Geometry: see drawing. Coordinates: mm, zero at the bounding-box minimum. A direction names the side the tool comes from. Give positions to 0.01 mm unless a question says otherwise; leave off trailing zeros. Order: outer loops, then holes, each group sorted by start corner. A loop starts at its lowest first (then second) coordinate and runs counter-clockwise, first axis right, second up. Notation, with made-up numbers: M 65,17.25 L 121,17.25 A22 cw 121,46.25 Z; hole C 29,-37.75 d11. An arc over 180 degrees is marked long. Return JSON: item names as keys, results as strings.
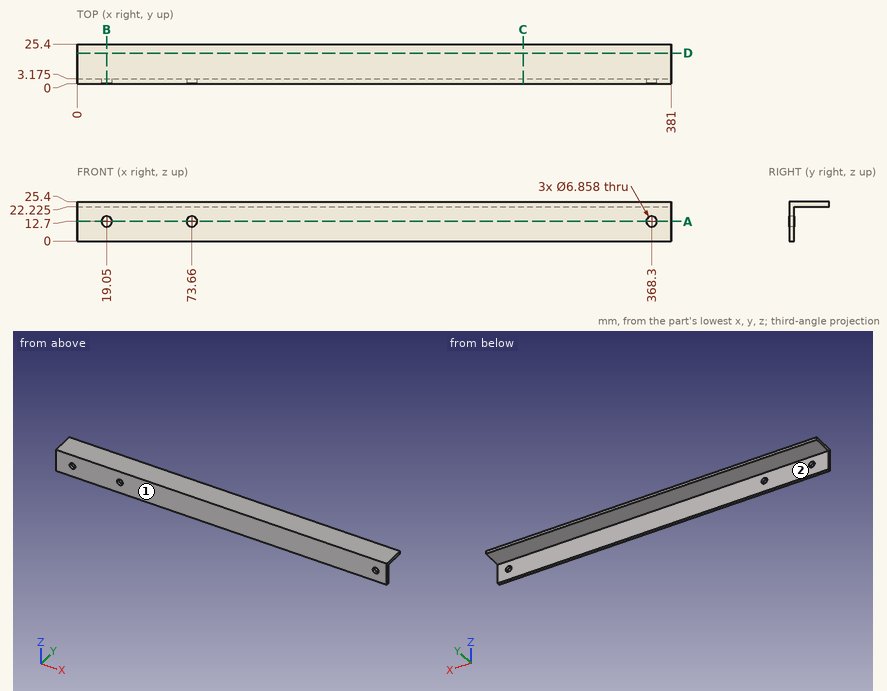
1. Set-up query: the marked faces 1 and 2. Return all of +Z, -Z, +X, -X, +Y, -Y with unobstructed straight access to the full face (end or side cutting, diameter ignored); none if empty.
Evaluation:
{"face 1": "+Z, -Z, +X, -X, -Y", "face 2": "-Z, +X, -X, +Y"}
2. Ray query, probe 1 along Z at (x, y) = (19.05, 2.2); probe 2 along Z at (x, y) = (284, 12.75) (3 decimals); probe 3 along X at (y, z) = (1.5, 14.25). Return the intervals inside material, ascending.
Evaluation:
{"probe 1": "z = 0 to 9.27, 16.13 to 25.4", "probe 2": "z = 22.225 to 25.4", "probe 3": "x = 0 to 15.99, 22.11 to 70.6, 76.72 to 365.24, 371.36 to 381"}
3. Section query C-C (x = 286). Return loops of the section in (y, z) (3 decimals), then the cut area to 3 significant figures.
Evaluation:
{"outline": "M 0,0 L 3.175,0 L 3.175,22.225 L 25.4,22.225 L 25.4,25.4 L 0,25.4 Z", "area": "151 mm^2"}
4. Section query B-B (x = 19.05). Return loops of the section in (y, z) (3 decimals), then the cut area to 3 significant figures.
Evaluation:
{"outline": "M 0,0 L 3.175,0 L 3.175,9.271 L 0,9.271 Z; M 0,16.129 L 3.175,16.129 L 3.175,22.225 L 25.4,22.225 L 25.4,25.4 L 0,25.4 Z", "area": "129 mm^2"}
5. Section query A-A (z = 12.7). Return loops of the section in (x, y) (3 decimals), then the cut area to 3 significant figures.
Evaluation:
{"outline": "M 0,0 L 15.621,0 L 15.621,3.175 L 0,3.175 Z; M 22.479,0 L 70.231,0 L 70.231,3.175 L 22.479,3.175 Z; M 77.089,0 L 364.871,0 L 364.871,3.175 L 77.089,3.175 Z; M 371.729,0 L 381,0 L 381,3.175 L 371.729,3.175 Z", "area": "1,140 mm^2"}
6. Section query D-D (y = 19.5). Return loops of the section in (x, z) (3 decimals), then the cut area to 3 significant figures.
Evaluation:
{"outline": "M 0,22.225 L 381,22.225 L 381,25.4 L 0,25.4 Z", "area": "1,210 mm^2"}
7. First-contact query: pin 1 (11 mm diameter, centred on x = 19.05, z = 12.7, fed in from +Y) (3 decimals); pin 2 (2 mm diameter, centred on x = 109, y = 12, fed in from -Z) (3 decimals). Flat tips, straight axial feed; report the tip coordinate or a pass-through.
Evaluation:
{"pin 1": "stops at y = 3.175", "pin 2": "stops at z = 22.225"}
